Can you work these out from the model? Positions are in its coordinate system, mm. Round coordinates to 2 decimals unless told otherwise and drop trailing zeros. Write each loop counter-clockwise with the first axis right and the second up, starting at its lowest first coordinate (ties: lowest second). Pieces come first, ordered by that corner, then holes. Notation, with made-up numbers: (56, -25.5) - (94, -25.5) arc R7 ccw to (94, -16.5) - close; hole circle Ø5 at (85, 37). An arc over 180 degrees is marked (long way). One line per item, written item: value. Start each with the question number.
(1) I want a section at A-A on x = -36. List the corners of the cut face in (y, z) for me, plus the area to 3 significant figures.
(2) I want a section at C-C on y = 4.5. List the corners of the cut face in (x, z) for me, plus the area to 3 significant figures.
(3) If I drill on L1, parallel to Y at x = 4.5, z = 42.5; L2, parallel to Z at x = 39, y = -2.5; L3, parallel to Y at x = 37.5, z = 7, over which ranges is the centre line in solid material (lowest first)? Write a range as from..to.
(4) I'm going to push flat-ended pins straight in: pin 1 Ø4 at (x, y) = (9.5, 16) entering from +Z; pin 2 Ø1.5 at (y, z) = (13.5, 51.5) entering from -X; pin 3 Ø6 at (x, y) = (-23, -25.5) entering from +Z; pin 4 Ø1.5 at (x, y) = (-34, -14) entering from +Z. Where does each tip first touch, or does it pass through?
(5) I want a section at B-B on z = 6. List the corners of the cut face in (x, y) for me, plus the area to 3 significant figures.
(6) I want a section at D-D on z = 34. List the corners of the cut face in (x, y) for me.
from build123d import *

# Parameters (mm, degrees)
F1_DEPTH = 63.5
F3_DEPTH = 107.692191


with BuildPart() as f1:
    # F0 (on Top) → F1 (new body)
    with BuildSketch(Plane.XY):
        Polygon((53.845596, 0), (53.845596, 34.127489), (-53.845596, 34.127489), (-53.845596, -34.127489), (28.818766, -34.127489), align=None)
    extrude(amount=F1_DEPTH)

    # F2 (on face) → F3 (cut, through all)
    with BuildSketch(Plane(origin=(-53.845596, 0, 0), x_dir=(0, -1, 0), z_dir=(-1, 0, 0))):
        Polygon((34.127489, 63.5), (-34.127489, 63.5), (34.127489, 22.182867), align=None)
    extrude(amount=-F3_DEPTH, mode=Mode.SUBTRACT)


solid = f1.part
Established:
1. outline: (-34.13, 0) - (34.13, 0) - (34.13, 63.5) - (-34.13, 22.18) - close
1. area: 2,920 mm2
2. outline: (-53.85, 0) - (53.85, 0) - (53.85, 45.57) - (-53.85, 45.57) - close
2. area: 4,910 mm2
3. L1: -0.56..34.13
3. L2: 0..41.33
3. L3: -22.29..34.13
4. pin 1: z = 53.74
4. pin 2: x = -53.85
4. pin 3: z = 29.22
4. pin 4: z = 34.82
5. outline: (-53.85, -34.13) - (28.82, -34.13) - (53.85, 0) - (53.85, 34.13) - (-53.85, 34.13) - close
5. area: 6,920 mm2
6. outline: (-53.85, -14.61) - (43.13, -14.61) - (53.85, 0) - (53.85, 34.13) - (-53.85, 34.13) - close
